Autodesk Inventor part; units mm, degrees
ref_plane "YZ Plane" through (0, 0, 0) normal (1, 0, 0) x (0, 1, 0)
ref_plane "XZ Plane" through (0, 0, 0) normal (0, 1, 0) x (-1, 0, 0)
ref_plane "XY Plane" through (0, 0, 0) normal (0, 0, 1) x (1, 0, 0)
sketch "Sketch1" plane through (0, 0, 0) normal (0, 0, 1) x (1, 0, 0)
  circle A0 centre (0, 0) radius 15
  circle A1 centre (16, 16) radius 1.5
  circle A2 centre (-16, 16) radius 1.5
  circle A3 centre (-16, -16) radius 1.5
  circle A4 centre (16, -16) radius 1.5
  line L0 (20, -18) -> (20, 18)
  line L1 (18, 20) -> (-18, 20)
  line L2 (-60.0198, 26.9978) -> (-59.9853, -20.0189)
  line L3 (-18, -20) -> (18, -20)
  line L4 (-57.0198, 30) -> (-15.022, 30)
  line L5 (-14.978, -30) -> (-56.9802, -30)
  line L6 (-59.9802, -27.0022) -> (-60.0198, 26.9978)
  arc A5 (-59.9802, -27.0022) -> (-56.9802, -30) centre (-56.9802, -27) ccw
  arc A6 (-57.0198, 30) -> (-60.0198, 26.9978) centre (-57.0198, 27) ccw
  line L7 (20, -18) -> (20, 18)
  line L8 (-14.978, -30) -> (20, -30)
  line L9 (20, -30) -> (20, -18)
  line L10 (20, -30) -> (-56.9802, -30)
  line L11 (-60.0198, -29) -> (-60.0198, 27)
  line L12 (-57.0198, 30) -> (20, 30)
  line L13 (20, 30) -> (20, -30)
  point P0 (0, 0)
  point P1 (-60.0198, 26.9811)
  point P2 (-59.978, -30)
  dimension "d16" = 3
  dimension "d17" = 3
  dimension "d26" = 30
  dimension "d27" = 60
  dimension "d29" = 45
  dimension "d30" = 45
  dimension "d31" = 60
  dimension "d32" = 79.9853
  dimension "d33" = 80.0198
extrude "Extrusion1" add sketch "Sketch1" along normal blind 2
fillet "Fillet1" radius 5 2 edges at (20, -30, 1) (20, 30, 1)
sketch "Sketch4" plane through (0, 0, 2) normal (0, 0, 1) x (1, 0, 0)
  line L0 (-21.95, -0.0183) -> (-57.05, -0.0183) construction
  line L1 (-25, 3.0317) -> (-54, 3.0317)
  line L2 (-54, -3.0683) -> (-25, -3.0683)
  arc A0 (-25, -3.0683) -> (-25, 3.0317) centre (-25, -0.0183) ccw
  arc A1 (-54, 3.0317) -> (-54, -3.0683) centre (-54, -0.0183) ccw
  circle A2 centre (0, 0) radius 15
  line L3 (-60.0198, 26.9978) -> (-59.9802, -27.0022)
  point P0 (0, 0)
  point P1 (-39.5, -0.0183)
  dimension "d34" = 6.1
  dimension "d35" = 25
  dimension "d36" = 6
extrude "Extrusion2" cut sketch "Sketch4" against normal through all contours A0 L2 A1 L1
sketch "Sketch5" plane through (0, 0, 2) normal (0, 0, 1) x (1, 0, 0)
  point P0 (0, 0)
sketch "Sketch6" plane through (0, 0, 2) normal (0, 0, 1) x (1, 0, 0)
  line L0 (15, 30) -> (-57.0198, 30)
  line L1 (7, 30) -> (-55, 30) construction
  line L2 (7, 34) -> (-55, 34)
  line L3 (-55, 26) -> (7, 26)
  arc A0 (7, 26) -> (7, 34) centre (7, 30) ccw
  arc A1 (-55, 34) -> (-55, 26) centre (-55, 30) ccw
  point P0 (0, 0)
  point P1 (-24, 30)
  dimension "d39" = 62
extrude "Extrusion3" cut sketch "Sketch6" against normal through all
ref_plane "Work Plane1" through (15, 0, 2) normal (0, 1, 0) x (1, 0, 0)
mirror "Mirror1" about plane through (15, 0, 2) normal (0, 1, 0) of "Extrusion3"
equation "\"d30\" = d29"
properties part number "X-motor-holder"
Input: part model. Units: mm. Frame: model coordinates. A direction names the side the tool comes from. Give positions to 0.01 mm unless a question says otherwise; leave off trailing zeros. Order: outer loops, then holes, each group sorted by start corner. A loop starts at its lowest first (then second) coordinate and runs counter-clockwise, first axis right, second up. Notation, with made-up numbers: (16, -2) - (25, -2) arc R19 ccw to (25, 14) - close; hole circle Ø7 at (56, 31.5). An arc over 180 degrees is marked (long way). Use a Markdown table: item, result.
(1) Pin query (flat end, axial travel): pin 1 (2.5 mm diameter, centred on x = -16, y = 16, fed in from +Z); pin 2 (0.6 mm diameter, centred on x = -14, z = 1, fed in from -Y); pin 3 (0.6 mm diameter, centred on x = -43.5, z = 1, fed in from +Y). Return the tip coordinate at first contact, or that it passes through.
Computed values:
| item | result |
|---|---|
| pin 1 | passes through |
| pin 2 | stops at y = -26 |
| pin 3 | stops at y = 26 |
(2) Section query D-D (y = 1). Output: boundary loops of the cut face in (x, z).
Computed values:
| item | result |
|---|---|
| outline | (-60, 0) - (-56.87, 0) - (-56.87, 2) - (-60, 2) - close; (-22.13, 0) - (-14.97, 0) - (-14.97, 2) - (-22.13, 2) - close; (14.97, 0) - (20, 0) - (20, 2) - (14.97, 2) - close |
(3) Draft query along Y for faces 1 (the flat face through (20, 0, 1)), 2 (the cylindrical face through (9.797, 27.141, 1.014)), 3 (the flat face through (-39, 3.032, 1)), 4 (the flat face through (-40, -3.068, 1)). Return one class per face: released by +Y, released by -Y, zero draft, split by the parting line, or undercut.
Computed values:
| item | result |
|---|---|
| face 1 | zero draft |
| face 2 | released by +Y |
| face 3 | undercut |
| face 4 | undercut |
(4) Section query C-C (x = -16). Output: boundary loops of the cut face in (y, z), then the cut area to 3 significant figures.
Computed values:
| item | result |
|---|---|
| outline | (-26, 0) - (-17.5, 0) - (-17.5, 2) - (-26, 2) - close; (-14.5, 0) - (14.5, 0) - (14.5, 2) - (-14.5, 2) - close; (17.5, 0) - (26, 0) - (26, 2) - (17.5, 2) - close |
| area | 92.0 mm2 |
(5) Section query A-A (x = -51.5). Output: boundary loops of the cut face in (y, z), then the cut area to 3 significant figures.
Computed values:
| item | result |
|---|---|
| outline | (-26, 0) - (-3.07, 0) - (-3.07, 2) - (-26, 2) - close; (3.03, 0) - (26, 0) - (26, 2) - (3.03, 2) - close |
| area | 91.8 mm2 |
(6) Section query B-B (z = 1.7). Output: boundary loops of the cut face in (x, y).
Computed values:
| item | result |
|---|---|
| outline | (-60.02, 27) - (-59.99, -20.02) - (-59.98, -27) arc R3 ccw to (-58.93, -29.28) arc R4 cw to (-55, -26) - (7, -26) arc R4 cw to (11, -30) - (15, -30) arc R5 ccw to (20, -25) - (20, 25) arc R5 ccw to (15, 30) - (11, 30) arc R4 cw to (7, 26) - (-55, 26) arc R4 cw to (-58.94, 29.31) arc R3 ccw to start; hole (-54, -3.07) - (-25, -3.07) arc R3.05 ccw to (-25, 3.03) - (-54, 3.03) arc R3.05 ccw to start; hole circle Ø3 at (-16, -16); hole circle Ø3 at (-16, 16); hole circle Ø30 at (0, 0); hole circle Ø3 at (16, -16); hole circle Ø3 at (16, 16) |
(7) Line query: line 1 (Y direction, x = -16, z = 0.5); line 2 (X direction, y = 0.5, z = 0.4); line 3 (Y direction, x = 16, z = 1.05). Output: solid intervals per line, ascending. Write a range as from..to.
Computed values:
| item | result |
|---|---|
| line 1 | y = -26..-17.5, -14.5..14.5, 17.5..26 |
| line 2 | x = -60..-57.01, -21.99..-14.99, 14.99..20 |
| line 3 | y = -29.9..-17.5, -14.5..14.5, 17.5..29.9 |
(8) Access query for faces 5 (the flat face through (13, -30, 1)), 6 (the cylindrical face through (-21.95, -0.09, 1.01)), 7 (the cylindrical face through (-57.6, 26.96, 1.01)), 8 (the flat face through (-24, -26, 1)). Directions: +Z, -Z, +X, -X, +Y, -Y. A direction counts if a zero-diameter tool reaches every point of the face in a straight line with its end or side. Return the directions, or none.
Computed values:
| item | result |
|---|---|
| face 5 | +Z, -Z, +X, -X, -Y |
| face 6 | +Z, -Z |
| face 7 | +Z, -Z, +Y |
| face 8 | +Z, -Z, -Y |
